Verification items for the finished model (mm, model axes). A direction names the side the tool comes from. Give positions to 0.01 mm unless a question says otherwise; leave off trailing zeros. Write each loop counter-clockwise with the first axis right and the second up, starting at its lowest first coordinate (ties: lowest second). Pieces come first, ordered by that corner, then holes. Notation, with made-up numbers: (70.25, 81) - (80.25, 81) arc R18 cw to (80.25, 99) - close; hole circle Ø8 at (-38.5, 29.25). An arc over 180 degrees is marked (long way). Put each result on its own line as item: value.
from build123d import *

# Parameters (mm, degrees)
REVOLVE1_ANGLE      = 60
SKETCH2_OUTSIDE_W   = 36.094
SKETCH2_OUTSIDE_H   = 57.312
SKETCH2_OUTSIDE_W_2 = 27.637577589
SKETCH2_OUTSIDE_H_2 = 30
CUT_EXTRUDE2_DEPTH  = 40
FILLET1_R           = 5
SKETCH3_R           = 1.75
CUT_EXTRUDE3_DEPTH  = 40


with BuildPart() as part:
    # Sketch1 → Revolve1 (revolve, symmetric)
    with BuildSketch(Plane.XY) as revolve1_sk:
        Polygon((30, 20), (30, 10.5), (24.5, 5), (24.5, 0), (44.5, 0), (44.5, 20), align=None)
    revolve(axis=Axis((0, 0, 0), (0, 1, 0)), revolution_arc=REVOLVE1_ANGLE / 2)
    revolve(revolve1_sk.sketch, axis=Axis((0, 0, 0), (0, -1, 0)), revolution_arc=REVOLVE1_ANGLE / 2)

    # Sketch2 outside → Cut-Extrude2 (cut)
    with BuildSketch(Plane(origin=(0, 0, 0), x_dir=(1, 0, 0), z_dir=(0, 1, 0))):
        with Locations((32.859, 0)):
            Rectangle(SKETCH2_OUTSIDE_W, SKETCH2_OUTSIDE_H)
        with Locations((25.681211205, 0)):
            Rectangle(SKETCH2_OUTSIDE_W_2, SKETCH2_OUTSIDE_H_2, mode=Mode.SUBTRACT)
    extrude(amount=CUT_EXTRUDE2_DEPTH, mode=Mode.SUBTRACT)

    # Fillet1
    fillet1_edges = [part.edges().sort_by_distance(p)[0] for p in [
        (39.5, 10, -15),
        (39.5, 10, 15),
    ]]
    fillet(fillet1_edges, radius=FILLET1_R)

    # Sketch3 → Cut-Extrude3 (cut)
    with BuildSketch(Plane(origin=(0, 20, 0), x_dir=(1, 0, 0), z_dir=(0, 1, 0))):
        with Locations(Location((34.5, -10, 0), (0, 0, 270))):
            Circle(SKETCH3_R)
        with Locations(Location((34.5, 10, 0), (0, 0, 270))):
            Circle(SKETCH3_R)
        with Locations(Location((34.5, 0, 0), (0, 0, 270))):
            Circle(SKETCH3_R)
    extrude(amount=-CUT_EXTRUDE3_DEPTH, mode=Mode.SUBTRACT)


solid = part.part
Q1. Section check A-A, the plane z = 0. Record the cut outline in (x, y).
Answers follow:
outline: (24.5, 0) - (32.75, 0) - (32.75, 20) - (30, 20) - (30, 10.5) - (24.5, 5) - close; (36.25, 0) - (39.5, 0) - (39.5, 20) - (36.25, 20) - close
Q2. Section check C-C, the plane x = 34. Record the cut outline in (y, z), plus the area to 3 significant figures.
Answers follow:
outline: (0, -15) - (20, -15) - (20, -11.68) - (0, -11.68) - close; (0, -8.32) - (20, -8.32) - (20, -1.68) - (0, -1.68) - close; (0, 1.68) - (20, 1.68) - (20, 8.32) - (0, 8.32) - close; (0, 11.68) - (20, 11.68) - (20, 15) - (0, 15) - close
area: 399 mm2
Q3. Scan lines: line 1 along X through (y, z) = (14, 0); line 2 along Z through (x, y) = (22.75, 6.5); line 3 along X through (y, z) = (15, 10). Record each from-to range of solid material in increasing order.
Answers follow:
line 1: x = 30 to 32.75, 36.25 to 39.5
line 2: z = -13.13 to -12.59, 12.59 to 13.13
line 3: x = 28.28 to 32.75, 36.25 to 39.5
Q4. Set-up check for faces 1 (the face through (30, 15, 0)), 2 (the face through (24.095, 4.157, 13.911)): record each of +Z, -Z, +X, -X, +Y, -Y from which the full face is reachable in a straight line by a thin tool's end or side.
Answers follow:
face 1: -X, +Y
face 2: +Z, -X, +Y, -Y
Q5. Go/stop test with flat-tipped pins: pin 1 Ø6 at (x, z) = (26, -3.5) entering from +Y; pin 2 Ø3 at (x, z) = (34.5, -10) entering from +Y; pin 3 Ø8 at (y, z) = (4.5, 9) entering from -X; pin 4 Ø10 at (x, z) = (24.5, 3) entering from +Y. Record where each tip stops, or that it passes through.
Answers follow:
pin 1: stops at y = 9.73
pin 2: passes through
pin 3: stops at x = 21.22
pin 4: stops at y = 10.18
Q6. Section check D-D, the plane y = 14. Record the cut outline in (x, z).
Answers follow:
outline: (25.98, -15) - (34.5, -15) arc R5 ccw to (39.5, -10) - (39.5, 10) arc R5 ccw to (34.5, 15) - (25.98, 15) arc R30 cw to start; hole circle Ø3.5 at (34.5, -10); hole circle Ø3.5 at (34.5, 0); hole circle Ø3.5 at (34.5, 10)
Q7. Section check B-B, the plane y = 2.75. Record the cut outline in (x, z).
Answers follow:
outline: (21.22, -12.25) - (25.98, -15) - (34.5, -15) arc R5 ccw to (39.5, -10) - (39.5, 10) arc R5 ccw to (34.5, 15) - (25.98, 15) - (21.22, 12.25) arc R24.5 cw to start; hole circle Ø3.5 at (34.5, -10); hole circle Ø3.5 at (34.5, 0); hole circle Ø3.5 at (34.5, 10)
Q8. Release check for a two-part mould opening along Z. For faces 3 (the face through (30, 0, 0)), 4 (the face through (30, 10, 15)), 5 (the face through (35.026, 10.14, 11.669)), 6 (the face through (24.095, 4.157, -13.911)) record: released by +Z, released by -Z, zero draft, split by the parting line, or undercut.
Answers follow:
face 3: zero draft
face 4: released by +Z
face 5: undercut
face 6: released by -Z
